Model file for the job. Use its own axes, mm. Give positions to 0.01 mm unless a question says otherwise; leave off trailing zeros. Write each loop counter-clockwise with the first axis right and the second up, starting at its lowest first coordinate (ties: lowest second). Pieces come first, ordered by that corner, then holes. Notation, with made-up numbers: M -36.5,55.25 L 7.5,55.25 A34 ccw 7.5,86.25 Z; hole C 9.25,26.25 d5. An arc over 180 degrees is marked long. Answer as a JSON object with one key per item and string values. Group by question number.
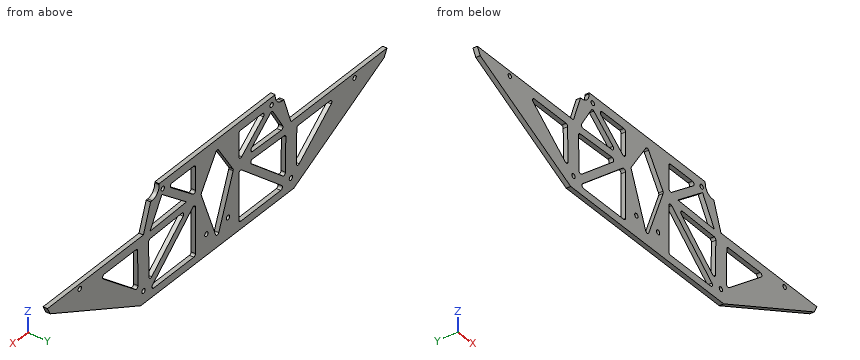
```python
from build123d import *

# Parameters (mm, degrees)
EXTRUDE_1_DEPTH     = 6
SKETCH_2_R          = 3
CUT_EXTRUDE_1_DEPTH = 318.409896722
FILLET_1_R          = 3


with BuildPart() as part:
    # Эскиз1 → Бобышка-Вытянуть1 (new body)
    with BuildSketch(Plane(origin=(0, 0, 0), x_dir=(1, 0, 0), z_dir=(0, 1, 0))):
        with BuildLine():
            Line((309.177837991, -19.526563843), (304.1208994, -9.869304954))
            Line((304.1208994, -9.869304954), (139.339108595, 71.568896564))
            Line((139.339108595, 71.568896564), (-139.339108595, 71.568896564))
            Line((-139.339108595, 71.568896564), (-304.1208994, -9.869304954))
            Line((-304.1208994, -9.869304954), (-309.177837991, -19.526563843))
            Line((-309.177837991, -19.526563843), (-134.367548184, -19.526563843))
            Line((-134.367548184, -19.526563843), (-121.255506601, -56.137850168))
            Line((-121.255506601, -56.137850168), (-118.625, -56.137850168))
            add(Edge.make_bspline(
                [(-118.625, -56.137850168), (-117.73604939, -56.137850168), (-116.863581866, -56.233656219), (-115.578458559, -56.514409609), (-115.154045806, -56.631020903), (-114.313330245, -56.91138161), (-113.900260231, -57.074299025), (-112.700337662, -57.62175838), (-111.944761063, -58.066913832), (-110.877012416, -58.853219635), (-110.532359667, -59.135456666), (-109.879727858, -59.72693005), (-109.259674848, -60.348234431), (-108.702715184, -61.027310664), (-108.177181377, -61.735162196), (-107.929156775, -62.105311768), (-107.245045383, -63.239220647), (-106.864936074, -64.029470546), (-106.249383942, -65.67531101), (-106.013919219, -66.536987879), (-105.703263791, -68.270165649), (-105.625, -69.14709382), (-105.625, -70.034522256)],
                knots=[0, 0, 0, 0, 0.125, 0.125, 0.1875, 0.1875, 0.25, 0.25, 0.375, 0.375, 0.4375, 0.4375, 0.5, 0.5625, 0.5625, 0.625, 0.625, 0.75, 0.75, 0.875, 0.875, 1, 1, 1, 1], degree=3))
            Line((-105.625, -70.034522256), (-105.625, -71.568896564))
            Line((-105.625, -71.568896564), (105.625, -71.568896564))
            Line((105.625, -71.568896564), (105.625, -70.034522256))
            add(Edge.make_bspline(
                [(105.625, -70.034522256), (105.625, -69.146188417), (105.703417019, -68.271043449), (105.934814701, -66.977461208), (106.031042325, -66.549478705), (106.262646487, -65.700098111), (106.398816423, -65.276664427), (106.863134882, -64.032516396), (107.243720136, -63.242761719), (107.92127714, -62.117712579), (108.165026803, -61.75269229), (108.68986891, -61.043508559), (108.97254159, -60.69784736), (109.860275675, -59.715540738), (110.508242307, -59.12685949), (111.565919809, -58.344904551), (111.932862686, -58.101210315), (112.6970874, -57.649589406), (113.090639287, -57.444106887), (114.289999629, -56.895653779), (115.12040105, -56.616320302), (116.41376972, -56.331041481), (116.854501373, -56.258404071), (117.736783928, -56.162064753), (118.179895928, -56.137850168), (118.625, -56.137850168)],
                knots=[0, 0, 0, 0, 0.125, 0.125, 0.1875, 0.1875, 0.25, 0.25, 0.375, 0.375, 0.4375, 0.4375, 0.5, 0.5, 0.625, 0.625, 0.6875, 0.6875, 0.75, 0.75, 0.875, 0.875, 0.9375, 0.9375, 1, 1, 1, 1], degree=3))
            Line((118.625, -56.137850168), (121.255506601, -56.137850168))
            Line((121.255506601, -56.137850168), (134.367548184, -19.526563843))
            Line((134.367548184, -19.526563843), (309.177837991, -19.526563843))
        make_face()
        Polygon((-214.327282353, -7.526563843), (-144.945354376, -7.526563843), (-144.232879574, 48.548456393), align=None, mode=Mode.SUBTRACT)
        Polygon((-124.234493737, 48.29436204), (-124.94696854, -7.780658197), (-55.587438417, -9.543471524), align=None, mode=Mode.SUBTRACT)
        Polygon((-39.584708108, 61.232071167), (-124.070110529, 61.232071167), (-39.584708108, -9.950190344), align=None, mode=Mode.SUBTRACT)
        Polygon((-29.584708108, -14.755399706), (0, -59.568896564), (29.584708108, -14.755399706), (0, 61.232071167), align=None, mode=Mode.SUBTRACT)
        Polygon((-90.997346953, -59.568896564), (-39.584708108, -59.568896564), (-39.584708108, -19.560609068), align=None, mode=Mode.SUBTRACT)
        Polygon((-99.853084476, -54.031919172), (-55.841512263, -19.540243327), (-122.220473813, -17.853182906), align=None, mode=Mode.SUBTRACT)
        Polygon((124.070110529, 61.232071167), (39.584708108, 61.232071167), (39.584708108, -9.950190344), align=None, mode=Mode.SUBTRACT)
        Polygon((124.94696854, -7.780658197), (124.234493737, 48.29436204), (55.587438417, -9.543471524), align=None, mode=Mode.SUBTRACT)
        Polygon((100.785410724, -54.522211893), (122.220473813, -17.853182906), (55.841512263, -19.540243327), align=None, mode=Mode.SUBTRACT)
        Polygon((90.997346953, -59.568896564), (39.584708108, -19.560609068), (39.584708108, -59.568896564), align=None, mode=Mode.SUBTRACT)
        Polygon((144.945354376, -7.526563843), (214.327282353, -7.526563843), (144.232879574, 48.548456393), align=None, mode=Mode.SUBTRACT)
    extrude(amount=EXTRUDE_1_DEPTH)

    # Эскиз2 → Вырез-Вытянуть1 (cut, through all)
    with BuildSketch(Plane(origin=(0, 6, 0), x_dir=(1, 0, 0), z_dir=(0, 1, 0))):
        with Locations(Location((-250.253196754, -12.871881409, 0), (0, 0, 270))):
            Circle(SKETCH_2_R)
        with Locations(Location((-134.151495051, 54.89026378, 0), (0, 0, 270))):
            Circle(SKETCH_2_R)
        with Locations(Location((-99.138834526, -61.401125149, 0), (0, 0, 270))):
            Circle(SKETCH_2_R)
        with Locations(Location((-19.792354054, 43.436505789, 0), (0, 0, 270))):
            Circle(SKETCH_2_R)
        with Locations(Location((19.792354054, 43.436505789, 0), (0, 0, 270))):
            Circle(SKETCH_2_R)
        with Locations(Location((99.138834526, -61.401125149, 0), (0, 0, 270))):
            Circle(SKETCH_2_R)
        with Locations(Location((134.151495051, 54.89026378, 0), (0, 0, 270))):
            Circle(SKETCH_2_R)
        with Locations(Location((250.253196754, -12.871881409, 0), (0, 0, 270))):
            Circle(SKETCH_2_R)
    extrude(amount=-CUT_EXTRUDE_1_DEPTH, mode=Mode.SUBTRACT)

    # Скругление1
    fillet_1_edges = [part.edges().sort_by_distance(p)[0] for p in [
        (-122.220473813, 3, 17.853182906),
        (-99.853084476, 3, 54.031919172),
        (-55.841512263, 3, 19.540243327),
        (39.584708108, 3, 9.950190344),
        (124.070110529, 3, -61.232071167),
        (39.584708108, 3, -61.232071167),
        (55.587438417, 3, 9.543471524),
        (124.94696854, 3, 7.780658197),
        (124.234493737, 3, -48.29436204),
        (39.584708108, 3, 59.568896564),
        (90.997346953, 3, 59.568896564),
        (39.584708108, 3, 19.560609068),
        (144.232879574, 3, -48.548456393),
        (144.945354376, 3, 7.526563843),
        (214.327282353, 3, 7.526563843),
        (-144.232879574, 3, -48.548456393),
        (-214.327282353, 3, 7.526563843),
        (-144.945354376, 3, 7.526563843),
        (-55.587438417, 3, 9.543471524),
        (-124.234493737, 3, -48.29436204),
        (-124.94696854, 3, 7.780658197),
        (-39.584708108, 3, 9.950190344),
        (-39.584708108, 3, -61.232071167),
        (-124.070110529, 3, -61.232071167),
        (0, 3, -61.232071167),
        (-29.584708108, 3, 14.755399706),
        (0, 3, 59.568896564),
        (29.584708108, 3, 14.755399706),
        (-39.584708108, 3, 19.560609068),
        (-90.997346953, 3, 59.568896564),
        (-39.584708108, 3, 59.568896564),
    ]]
    fillet(fillet_1_edges, radius=FILLET_1_R)


solid = part.part
```
Q1. Slice it at B-B, the plane z = -32. Count the separate pieces of the cut face and the enclosed holes in it, then the cut area to 3 significant figures.
Q2. Slice it at A-A, the plane x = 199. Write the cut outline in (y, z), then the cut area to 3 significant figures.
Q3. Drop flat-ended pins along their axis: P1, Ø1, axis at y = 1, z = 8.5, coming from the +X side; P2, Ø3, axis at x = 174, y = 2, coming from the +Z side; P3, Ø8, axis at x = -99.14, z = 61.4, coming from the +Y side; P4, Ø1.5, axis at x = -214, y = 1, coming from the -Z side. Give the stop position or say it passes through.
Q4. Wall check: L1, parallel to Z at x = -66, y = 5.25; L2, parallel to X at y = 2, z = 24; L3, parallel to Z at x = -73, y = 3.5. Give the ranges that are in metal, low to high.
Q5. Slice it at C-C, the plane x = -169.5. Write the cut outline in (y, z), then the cut area to 3 significant figures.
Solved:
{
 "1": {"separate pieces": "8", "enclosed holes": "0", "area": "1,420 mm²"},
 "2": {"outline": "M 0,-42.08 L 6,-42.08 L 6,-4.74 L 0,-4.74 Z; M 0,7.53 L 6,7.53 L 6,19.53 L 0,19.53 Z", "area": "296 mm²"},
 "3": {"P1": "stops at x = 302.36", "P2": "stops at z = 19.53", "P3": "stops at y = 6", "P4": "stops at z = -35.04"},
 "4": {"L1": "z = -71.57 to -61.23, -12.31 to 0.77, 9.28 to 19.28, 27.5 to 40.12, 59.57 to 71.57", "L2": "x = -132.77 to -118.42, -61.77 to -45.29, -40.11 to -23.48, 23.48 to 40.11, 45.29 to 61.57, 118.63 to 132.77", "L3": "z = -71.57 to -61.23, -18.2 to -5.13, 9.1 to 19.1, 32.99 to 45.56, 59.57 to 71.57"},
 "5": {"outline": "M 0,-56.66 L 6,-56.66 L 6,-28.33 L 0,-28.33 Z; M 0,7.53 L 6,7.53 L 6,19.53 L 0,19.53 Z", "area": "242 mm²"}
}
